Geometry: final body of the model. Coordinates: model frame, mm. Face numbers are marked on the shaded views. A direction names the side the tool comes from. Round coordinates to 2 decimals unless told otherwise and drop trailing zeros. Order: outer loops, then holes, each group sorted by start corner. A loop starts at its lowest first (then second) coordinate and runs counter-clockwise, first axis right, second up. Notation, with made-up numbers: M 5.5,82 L 53.5,82 A23 cw 53.5,111 Z; hole C 62.25,28 d11. An arc over 180 degrees is marked long. Put each result on its own line as item: value. Start each with the question number.
1) Section D-D, the plane x = -17. Return loops of the section in (y, z).
2) Draft query along X for the marked faces 1, 2, 3 and 4. Return one class per face: pulls with the +X half, pulls with the -X half, needs draft (parallel to the pull), parting line crosses it, or undercut.
3) First-contact query: P1, Ø2, axis at x = 12.5, y = -7.5, coming from the -Z side; P2, Ø1, axis at y = -5.5, z = 25, coming from the +X side; P3, Ø1.5, axis at x = -11.5, z = 4, coming from the +Y side; P4, Ø2, axis at y = -3, z = -18.5, coming from the -X side. Flat tips, straight axial feed; report the tip coordinate or a pass-through.
4) Section B-B, the plane x = 0. Return loops of the section in (y, z).
5) Material intervals for probe 1 along Z at (x, y) = (18.5, -4); probe 2 along Z at (x, y) = (-26.5, -10.75); probe 3 along X at (y, z) = (-8.5, 4), sorted ascending. Write a range as [from, to].
6) Section A-A, the plane z = 0. Return loops of the section in (x, y), then the cut area to 3 significant figures.
7) Access query for the marked faces 5, 6, 7, 8 and 9. Directions: +Z, -Z, +X, -X, +Y, -Y. A direction counts if a zero-diameter tool reaches every point of the face in a straight line with its end or side. Return the directions, or none.
8) Section C-C, the plane y = -4.75. Return loops of the section in (x, z).
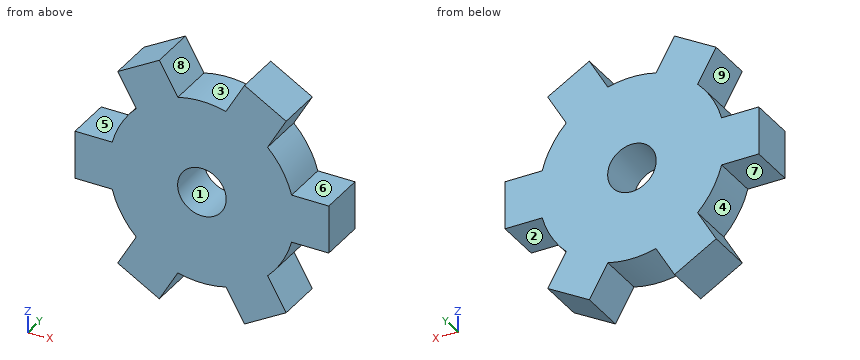
from build123d import *

# Parameters (mm, degrees)
F0_R     = 25.4
F1_DEPTH = 12.7
F3_DEPTH = 12.7
F5_COUNT = 6
F6_R     = 6.637445
F7_DEPTH = 12.701


with BuildPart() as f1:
    # F0 (on Front) → F1 (new body)
    with BuildSketch(Plane.XZ):
        Circle(F0_R)
    extrude(amount=F1_DEPTH)

    # F2 (on face) → F3 (join)
    with BuildSketch(Plane.XZ.offset(12.7)):
        Polygon((24.534516, 0), (0, 0), (24.534516, -6.574004), align=None)
        Polygon((24.534516, 6.574004), (0, 0), (24.534516, 0), align=None)
        with BuildLine():
            Line((24.534516, 6.574004), (24.534516, 0))
            Line((24.534516, 0), (25.4, 0))
            ThreePointArc((25.4, 0), (25.182699, 3.315365), (24.534516, 6.574004))
        make_face()
        with BuildLine():
            Line((25.4, 0), (24.534516, 0))
            Line((24.534516, 0), (24.534516, -6.574004))
            ThreePointArc((24.534516, -6.574004), (25.182699, -3.315365), (25.4, 0))
        make_face()
        with BuildLine():
            ThreePointArc((25.4, 0), (25.182699, -3.315365), (24.534516, -6.574004))
            Line((24.534516, -6.574004), (34.694516, -6.574004))
            Line((34.694516, -6.574004), (34.694516, 6.574004))
            Line((34.694516, 6.574004), (24.534516, 6.574004))
            ThreePointArc((24.534516, 6.574004), (25.182699, 3.315365), (25.4, 0))
        make_face()
    extrude(amount=-F3_DEPTH)

    # F5: F1 ×6 about axis
    f5_axis = Axis((0, 32.601867, 0), (0, 1, 0))


with BuildPart() as f1_1:
    add(f1.part)
    for i in range(1, F5_COUNT):
        add(f1.part.rotate(f5_axis, i * 360 / F5_COUNT))

    # F6 (on face) → F7 (cut, through all)
    with BuildSketch(Plane.XZ.offset(12.7)):
        Circle(F6_R)
    extrude(amount=-F7_DEPTH, mode=Mode.SUBTRACT)


solid = f1_1.part
Result sheet:
1. outline: M -12.7,-30.25 L 0,-30.25 L 0,30.25 L -12.7,30.25 Z
2. face 1: undercut
2. face 2: needs draft
2. face 3: undercut
2. face 4: pulls with the -X half
3. P1: stops at z = -33.33
3. P2: stops at x = 22.31
3. P3: stops at y = 0
3. P4: stops at x = -18.85
4. outline: M -12.7,-25.4 L 0,-25.4 L 0,-6.64 L -12.7,-6.64 Z; M -12.7,6.64 L 0,6.64 L 0,25.4 L -12.7,25.4 Z
5. probe 1: z = [-29.38, -18.89], [-17.4, 17.4], [18.89, 29.38]
5. probe 2: z = [-6.57, 6.57]
5. probe 3: x = [-34.69, -5.3], [5.3, 34.69]
6. outline: M -34.69,-12.7 L -6.64,-12.7 L -6.64,0 L -34.69,0 Z; M 6.64,-12.7 L 34.69,-12.7 L 34.69,0 L 6.64,0 Z
6. area: 713 mm2
7. face 5: +Z, -X, +Y, -Y
7. face 6: +Z, +X, +Y, -Y
7. face 7: -Z, -X, +Y, -Y
7. face 8: +Z, +Y, -Y
7. face 9: -X, +Y, -Y
8. outline: M -34.69,-6.57 L -24.53,-6.57 A25.4 ccw -17.96,-17.96 L -23.04,-26.76 L -11.65,-33.33 L -6.57,-24.53 A25.4 ccw 6.57,-24.53 L 11.65,-33.33 L 23.04,-26.76 L 17.96,-17.96 A25.4 ccw 24.53,-6.57 L 34.69,-6.57 L 34.69,6.57 L 24.53,6.57 A25.4 ccw 17.96,17.96 L 23.04,26.76 L 11.65,33.33 L 6.57,24.53 A25.4 ccw -6.57,24.53 L -11.65,33.33 L -23.04,26.76 L -17.96,17.96 A25.4 ccw -24.53,6.57 L -34.69,6.57 Z; hole C 0,0 d13.27
